Here's how the part is built. I have some questions about the finished solid (model axes, mm). Round coordinates to 2 decimals unless told otherwise and drop trailing zeros. Order: outer loops, then holes, each group sorted by start corner. A loop starts at its lowest first (then second) coordinate and runs counter-clockwise, first axis right, second up. Notation, with made-up numbers: M 3,80 L 8,80 A22 ccw 8,117 Z; hole C -11.5,2 d7. An arc over 180 degrees is marked long. Answer as CSV lines item,"result". Start each with the question number.
```python
from build123d import *

# Parameters (mm, degrees)
SKETCH1_W           = 350
SKETCH1_H           = 200
BOSS_EXTRUDE1_DEPTH = 3
SKETCH2_OUTSIDE_W   = 432.624
SKETCH2_OUTSIDE_H   = 282.624
SKETCH2_OUTSIDE_R   = 1.7
CUT_EXTRUDE1_DEPTH  = 10


with BuildPart() as part:
    # Sketch1 → Boss-Extrude1 (new body)
    with BuildSketch(Plane(origin=(0, 0, 0), x_dir=(1, 0, 0), z_dir=(0, 1, 0))):
        with Locations((175, 100)):
            Rectangle(SKETCH1_W, SKETCH1_H)
    extrude(amount=BOSS_EXTRUDE1_DEPTH)

    # Sketch2 outside → Cut-Extrude1 (cut)
    with BuildSketch(Plane(origin=(0, 3, 0), x_dir=(1, 0, 0), z_dir=(0, 1, 0))):
        with Locations((175, 100)):
            Rectangle(SKETCH2_OUTSIDE_W, SKETCH2_OUTSIDE_H)
        with BuildLine():
            Line((23.784579293, 37.646381187), (23.784579293, 167.845841187))
            ThreePointArc((23.784579293, 167.845841187), (25.834831825, 172.795588656), (30.784579293, 174.845841187))
            Line((30.784579293, 174.845841187), (318.483929293, 174.845841187))
            ThreePointArc((318.483929293, 174.845841187), (323.433676762, 172.795588656), (325.483929293, 167.845841187))
            Line((325.483929293, 167.845841187), (325.483929293, 37.646381187))
            ThreePointArc((325.483929293, 37.646381187), (323.433676762, 32.696633719), (318.483929293, 30.646381187))
            Line((318.483929293, 30.646381187), (30.784579293, 30.646381187))
            ThreePointArc((30.784579293, 30.646381187), (25.834831825, 32.696633719), (23.784579293, 37.646381187))
        make_face(mode=Mode.SUBTRACT)
        with Locations((303.284579293, 34.646381187)):
            Circle(SKETCH2_OUTSIDE_R)
        with Locations((217.284579293, 34.396381187)):
            Circle(SKETCH2_OUTSIDE_R)
        with Locations((45.284579293, 34.396381187)):
            Circle(SKETCH2_OUTSIDE_R)
        with Locations((131.284579293, 34.396381187)):
            Circle(SKETCH2_OUTSIDE_R)
        with Locations((303.284579293, 171.095841187)):
            Circle(SKETCH2_OUTSIDE_R)
        with Locations((217.284579293, 170.845841187)):
            Circle(SKETCH2_OUTSIDE_R)
        with Locations((45.284579293, 170.845841187)):
            Circle(SKETCH2_OUTSIDE_R)
        with Locations((131.284579293, 170.845841187)):
            Circle(SKETCH2_OUTSIDE_R)
        with BuildLine():
            Line((33.284579293, 167.345841187), (315.983929293, 167.345841187))
            ThreePointArc((315.983929293, 167.345841187), (317.398142856, 166.76005475), (317.983929293, 165.345841187))
            Line((317.983929293, 165.345841187), (317.983929293, 40.146381187))
            ThreePointArc((317.983929293, 40.146381187), (317.398142856, 38.732167625), (315.983929293, 38.146381187))
            Line((315.983929293, 38.146381187), (33.284579293, 38.146381187))
            ThreePointArc((33.284579293, 38.146381187), (31.870365731, 38.732167625), (31.284579293, 40.146381187))
            Line((31.284579293, 40.146381187), (31.284579293, 165.345841187))
            ThreePointArc((31.284579293, 165.345841187), (31.870365731, 166.76005475), (33.284579293, 167.345841187))
        make_face()
    extrude(amount=-CUT_EXTRUDE1_DEPTH, mode=Mode.SUBTRACT)


solid = part.part
```
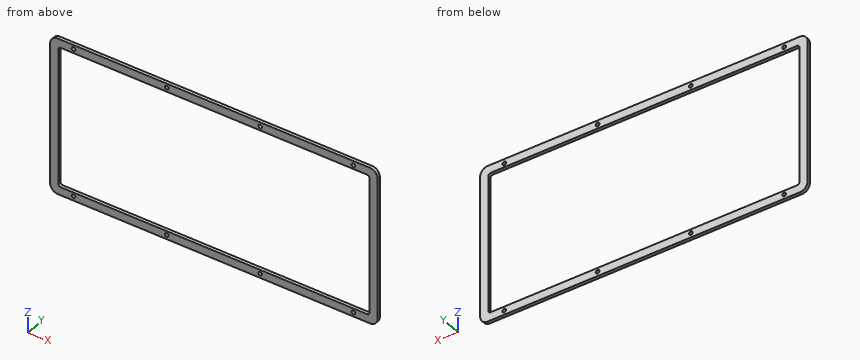
Item 1: If I drill on line 1 along Z through (x, y) = (284, 1.9); line 2 along X through (y, z) = (1.3, -41); line 3 along X through (y, z) = (0.75, -166), over which ranges is the centre line in solid material (lowest first)?
Item 2: If we section it at B-B on x = 242: Please give me the cut outline in (y, z), and give its area (3 significant figures).
Item 3: If we section it at C-C on y = 2.4: Count the separate pieces of the cut face and the enclosed holes in it, and give its area (3 significant figures).
Item 4: If we section it at A-A on z = -152.5: Please give me the cut outline in (x, y), and give its area (3 significant figures).
Geometry says:
1,line 1,"-174.85 to -167.35, -38.15 to -30.65"
1,line 2,"23.78 to 31.28, 317.98 to 325.48"
1,line 3,"23.78 to 31.39, 317.87 to 325.48"
2,outline,"M 0,-174.85 L 3,-174.85 L 3,-167.35 L 0,-167.35 Z; M 0,-38.15 L 3,-38.15 L 3,-30.65 L 0,-30.65 Z"
2,area,"45.0 mm²"
3,separate pieces,"1"
3,enclosed holes,"9"
3,area,"6,350 mm²"
4,outline,"M 23.78,0 L 31.28,0 L 31.28,3 L 23.78,3 Z; M 317.98,0 L 325.48,0 L 325.48,3 L 317.98,3 Z"
4,area,"45.0 mm²"
